Design review of the part built by this model. Coordinates are the model's own, in mm. Face numbers are marked on the shaded views. A direction names the side the tool comes from. Give positions to 0.01 mm unless a question says otherwise; leave off trailing zeros. Order: outer loops, then holes, each group sorted by start corner. A loop starts at its lowest first (then second) coordinate and runs counter-clockwise, first axis right, second up. Notation, with made-up numbers: (-17.5, -10.75) -> (-5.5, -10.75) arc R24 ccw to (-5.5, 1.25) -> close; hole circle Ø9 at (-24.5, 13). An arc over 180 degrees is marked (long way). Return JSON: item names as keys, results as strings.
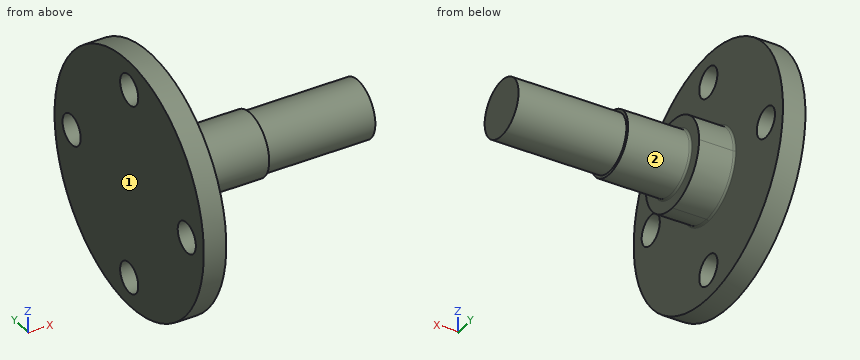
```python
from build123d import *

# Parameters (mm, degrees)
SKETCH1_W                = 120
SKETCH1_H                = 34
BOSS_EXTRUDE1_DEPTH      = 5
BOSS_EXTRUDE2_DEPTH      = 4
SKETCH3_R                = 3.5
BOSS_EXTRUDE3_DEPTH      = 19
SKETCH4_R                = 3.5
SKETCH4_R_2              = 3.175
CUT_EXTRUDE1_DEPTH       = 12
FILLET1_R                = 0.2
SKETCH5_W                = 120
SKETCH5_H                = 34
SKETCH5_R                = 14
CUT_EXTRUDE2_DEPTH       = 6
M3_CLEARANCE_HOLE1_D     = 3.4
M3_CLEARANCE_HOLE1_DEPTH = 15
M3_CLEARANCE_HOLE1_TIP   = 1.021463052
SKETCH9_W                = 2.5
SKETCH9_H                = 28
CUT_EXTRUDE6_DEPTH       = 29


with BuildPart() as part:
    # Sketch1 → Boss-Extrude1 (new body)
    with BuildSketch(Plane(origin=(0, 0, 0), x_dir=(0, 0, -1), z_dir=(1, 0, 0))):
        with Locations((-60, 17)):
            Rectangle(SKETCH1_W, SKETCH1_H)
    extrude(amount=BOSS_EXTRUDE1_DEPTH)

    # Sketch2 → Boss-Extrude2 (add)
    with BuildSketch(Plane(origin=(5, 0, 0), x_dir=(0, 0, -1), z_dir=(1, 0, 0))):
        with BuildLine():
            ThreePointArc((-55, 17), (-56.464466094, 20.535533906), (-60, 22))
            Line((-60, 22), (-60, 12))
            ThreePointArc((-60, 12), (-56.464466094, 13.464466094), (-55, 17))
        make_face()
        with BuildLine():
            Line((-60, 12), (-60, 22))
            ThreePointArc((-60, 22), (-65, 17), (-60, 12))
        make_face()
    extrude(amount=BOSS_EXTRUDE2_DEPTH)

    # Sketch3 → Boss-Extrude3 (add)
    with BuildSketch(Plane(origin=(9, 0, 0), x_dir=(0, 0, -1), z_dir=(1, 0, 0))):
        with Locations((-60, 17)):
            Circle(SKETCH3_R)
    extrude(amount=BOSS_EXTRUDE3_DEPTH)

    # Sketch4 → Cut-Extrude1 (cut)
    with BuildSketch(Plane(origin=(28, 0, 0), x_dir=(0, 0, -1), z_dir=(1, 0, 0))):
        with Locations((-60, 17)):
            Circle(SKETCH4_R)
        with Locations((-60, 17)):
            Circle(SKETCH4_R_2, mode=Mode.SUBTRACT)
    extrude(amount=-CUT_EXTRUDE1_DEPTH, mode=Mode.SUBTRACT)

    # Fillet1
    fillet1_edges = [part.edges().sort_by_distance(p)[0] for p in [
        (5, 12, 60),
        (9, 17, 63.5),
    ]]
    fillet(fillet1_edges, radius=FILLET1_R)

    # Sketch5 → Cut-Extrude2 (cut, through all)
    with BuildSketch(Plane(origin=(5, 0, 0), x_dir=(0, 0, -1), z_dir=(1, 0, 0))):
        with Locations((-60, 17)):
            Rectangle(SKETCH5_W, SKETCH5_H)
        with Locations((-60, 17)):
            Circle(SKETCH5_R, mode=Mode.SUBTRACT)
    extrude(amount=-CUT_EXTRUDE2_DEPTH, mode=Mode.SUBTRACT)

    # M3 Clearance Hole1
    with Locations(Plane(origin=(5, 0, 0), x_dir=(0, 0, -1), z_dir=(1, 0, 0))):
        with Locations((-60, 27.8), (-49.2, 17), (-60, 6.2), (-70.8, 17)):
            Hole(M3_CLEARANCE_HOLE1_D / 2, depth=M3_CLEARANCE_HOLE1_DEPTH)
            with Locations((0, 0, -(M3_CLEARANCE_HOLE1_DEPTH + M3_CLEARANCE_HOLE1_TIP / 2))):  # 118° drill point
                Cone(0, M3_CLEARANCE_HOLE1_D / 2, M3_CLEARANCE_HOLE1_TIP, mode=Mode.SUBTRACT)

    # Sketch9 → Cut-Extrude6 (cut, through all)
    with BuildSketch(Plane(origin=(0, 0, 46), x_dir=(-1, 0, 0), z_dir=(0, 0, -1))):
        with Locations((-1.25, 17)):
            Rectangle(SKETCH9_W, SKETCH9_H)
    extrude(amount=-CUT_EXTRUDE6_DEPTH, mode=Mode.SUBTRACT)


solid = part.part
```
Item 1: Add section A-A (z = 70.8). Give the boundary of the cut face in (x, y).
Result set:
{"outline": "(2.5, 8.09) -> (5, 8.09) -> (5, 15.3) -> (2.5, 15.3) -> close; (2.5, 18.7) -> (5, 18.7) -> (5, 25.91) -> (2.5, 25.91) -> close"}
Item 2: Add section B-B (y = 27.8). Give the boundary of the cut face in (x, z), plus the area to 3 significant figures.
Result set:
{"outline": "(2.5, 51.09) -> (5, 51.09) -> (5, 58.3) -> (2.5, 58.3) -> close; (2.5, 61.7) -> (5, 61.7) -> (5, 68.91) -> (2.5, 68.91) -> close", "area": "36.0 mm^2"}
Item 3: Machinability: for the marked faces 1 and 2, which of the approach directions +Z, -Z, +X, -X, +Y, -Y give a long, thin tool a straight path to every point of the face, cutting with its end or side? Answer none if there is none.
Result set:
{"face 1": "+Z, -Z, -X, +Y, -Y", "face 2": "+X"}
Item 4: Wall thickness on L1, parallel to Y at x = 3.85, z = 60; L2, parallel to X at y = 10.75, z = 60.5; L3, parallel to X at y = 20.75, z = 61.5: over which ranges is each line inside the solid? List them lowest first. Write a range as [from, to].
Result set:
{"L1": "y = [3, 4.5], [7.9, 26.1], [29.5, 31]", "L2": "x = [2.5, 5]", "L3": "x = [2.5, 9]"}
Item 5: Add section C-C (x = 21.25). Give the boundary of the cut face in (y, z) (3 decimals), plus the area to 3 significant figures.
Result set:
{"outline": "circle Ø6.35 at (17, 60)", "area": "31.7 mm^2"}
Item 6: For pin 1 (6 mm diameter, centred on x = 11, z = 57.5, fed in from +Y); pin 2 (12 mm diameter, centred on x = 12, y = 10, fed in from -Z); pin 3 (5.5 mm diameter, centred on y = 17, z = 70.8, fed in from -X); pin 4 (5.5 mm diameter, centred on y = 27.8, z = 60, fed in from +X), all flat-tipped, find the tip position at first contact; note any pin that passes through.
Result set:
{"pin 1": "stops at y = 21.99", "pin 2": "stops at z = 55.34", "pin 3": "stops at x = 2.5", "pin 4": "stops at x = 5"}
Item 7: Add section D-D (z = 53). Give the boundary of the cut face in (x, y), plus the area to 3 significant figures.
Result set:
{"outline": "(2.5, 4.88) -> (5, 4.88) -> (5, 29.12) -> (2.5, 29.12) -> close", "area": "60.6 mm^2"}
